Can you work these out from the model? Positions are in its coordinate system, mm. Give positions to 0.01 mm unless a question says otherwise; leave off trailing zeros. Use one line per item in the form item = value. Start each with the question number.
1. I want a section at A-A, the plane y = 13.5. Count the separate pieces of the cut face and the enclosed holes in it, and give its area (3 significant figures).
2. I need wall thicknesses on L1, parallel to Y at x = 405, z = 231.5 (3 decimals). Which ranges of the line are inside material? Lowest first, please.
3. Will this pin go through, and if not, where does the flat tip stop? P1, Ø9.5, axis at x = 252.5, z = 147.5, coming from the +Y side (3 decimals).
```python
from build123d import *

# Parameters (mm, degrees)
SKETCH1_W          = 1428.75
SKETCH1_H          = 762
BOARD_DEPTH        = 19.05
SKETCH9_W          = 19.05
SKETCH9_H          = 9.525
CUT_EXTRUDE1_DEPTH = 1479.800346565
LPATTERN1_COUNT    = 7
LPATTERN1_PITCH    = 88.9


with BuildPart() as part:
    # Sketch1 → Board (new body)
    with BuildSketch(Plane(origin=(0, 0, 0), x_dir=(1, 0, 0), z_dir=(0, 1, 0))):
        Rectangle(SKETCH1_W, SKETCH1_H)
    extrude(amount=BOARD_DEPTH)

    # Sketch9 → Cut-Extrude1 (cut, through all)
    with BuildSketch(Plane.ZY.offset(714.375)):
        with Locations((327.025, 14.2875)):
            Rectangle(SKETCH9_W, SKETCH9_H)
    cut_extrude1 = extrude(amount=-CUT_EXTRUDE1_DEPTH, mode=Mode.SUBTRACT)

    # LPattern1: Cut-Extrude1 ×7
    with Locations(*[(0, 0, -i * LPATTERN1_PITCH) for i in range(1, LPATTERN1_COUNT)]):
        add(cut_extrude1, mode=Mode.SUBTRACT)


solid = part.part
```
Check result:
q1.separate_pieces = 8
q1.enclosed_holes = 0
q1.area = 898,000 mm2
q2.L1 = 0 to 9.525
q3.P1 = 9.525
